```python
from build123d import *

# Parameters (mm, degrees)
F0_W     = 230.405122
F0_H     = 95.70128
F1_DEPTH = 25.4


with BuildPart() as f1:
    # F0 (on Front) → F1 (new body)
    with BuildSketch(Plane.XZ):
        Rectangle(F0_W, F0_H)
        Polygon((-70.301281, -22.45064), (-89.802561, -22.45064), (-89.802561, 2.94936), (-89.802561, 22.45064), (-70.301281, 22.45064), (-44.901281, 22.45064), (-19.501281, 22.45064), (19.501281, 22.45064), (44.901281, 22.45064), (70.301281, 22.45064), (89.802561, 22.45064), (89.802561, 2.94936), (89.802561, -22.45064), (64.402561, -22.45064), (25.4, -22.45064), (0, -22.45064), (-25.4, -22.45064), (-64.402561, -22.45064), align=None, mode=Mode.SUBTRACT)
        Polygon((-70.301281, 22.45064), (-70.301281, -22.45064), (-64.402561, -22.45064), (-44.901281, -2.94936), (-44.901281, 22.45064), align=None)
        Polygon((-44.901281, 22.45064), (-44.901281, -2.94936), (-25.4, -22.45064), (0, -22.45064), (0, 2.94936), (-19.501281, 22.45064), align=None)
        Polygon((0, 2.94936), (0, -22.45064), (25.4, -22.45064), (44.901281, -2.94936), (44.901281, 22.45064), (19.501281, 22.45064), align=None)
        Polygon((44.901281, 22.45064), (44.901281, -2.94936), (64.402561, -22.45064), (89.802561, -22.45064), (89.802561, 2.94936), (70.301281, 22.45064), align=None)
    extrude(amount=F1_DEPTH)


solid = f1.part
```
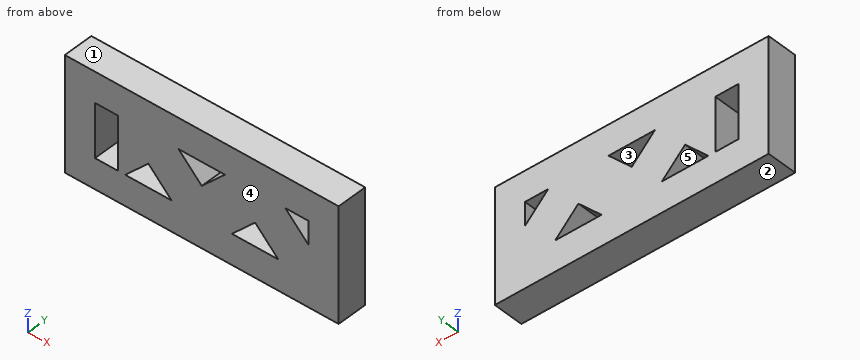
Geometry: final body of the model. Coordinates: model frame, mm. Face numbers are marked on the shaded views. A direction names the side the tool comes from. Round coordinates to 2 decimals unless told otherwise and drop trailing zeros. Order: outer loops, then holes, each group sorted by start corner. A loop starts at its lowest first (then second) coordinate and runs counter-clockwise, first axis right, second up. Notation, with made-up numbers: M 77,18.5 L 102,18.5 A17 ccw 102,37.5 Z; hole C 37.5,76.5 d6. An arc over 180 degrees is marked long. One line per item, written item: value.
(1) Cut plane D-D (x = -7). Return the cut outline in (y, z), and give its area (3 significant figures).
Result sheet:
outline: M -25.4,-47.85 L 0,-47.85 L 0,9.95 L -25.4,9.95 Z; M -25.4,22.45 L 0,22.45 L 0,47.85 L -25.4,47.85 Z
area: 2,110 mm2
(2) Pull-direction query (Z, two-part tool) for the marked faces 1, 2 and 3; classes: pulls with the +Z half, pulls with the -Z half, needs draft (parallel to the pull), parting line crosses it, or undercut.
Result sheet:
face 1: pulls with the +Z half
face 2: pulls with the -Z half
face 3: undercut
(3) Cut plane C-C (z = 10). Return the cut outline in (x, y).
Result sheet:
outline: M -115.2,-25.4 L -89.8,-25.4 L -89.8,0 L -115.2,0 Z; M -70.3,-25.4 L -7.05,-25.4 L -7.05,0 L -70.3,0 Z; M 7.05,-25.4 L 82.75,-25.4 L 82.75,0 L 7.05,0 Z; M 89.8,-25.4 L 115.2,-25.4 L 115.2,0 L 89.8,0 Z
(4) Cut plane B-B (y = -21). Return the cut outline in (x, z).
Result sheet:
outline: M -115.2,-47.85 L 115.2,-47.85 L 115.2,47.85 L -115.2,47.85 Z; hole M -89.8,-22.45 L -70.3,-22.45 L -70.3,22.45 L -89.8,22.45 Z; hole M -64.4,-22.45 L -25.4,-22.45 L -44.9,-2.95 Z; hole M -19.5,22.45 L 0,2.95 L 19.5,22.45 Z; hole M 25.4,-22.45 L 64.4,-22.45 L 44.9,-2.95 Z; hole M 70.3,22.45 L 89.8,2.95 L 89.8,22.45 Z
(5) Line query: probe 1 along X at (y, z) = (-20.5, -2.5); probe 2 along Z at (x, y) = (-76, -11.5); probe 3 along X at (y, z) = (-2.5, 10.5). Output: solid intervals per line, ascending. Write a range as [from, to].
Result sheet:
probe 1: [-115.2, -89.8], [-70.3, 115.2]
probe 2: [-47.85, -22.45], [22.45, 47.85]
probe 3: [-115.2, -89.8], [-70.3, -7.55], [7.55, 82.25], [89.8, 115.2]
(6) Reachability of the marked faces 4 and 5 from +Z, -Z, +X, -X, +Y, -Y: full face, straight path, thin tool, end or side. Return the list, or none.
Result sheet:
face 4: +Z, -Z, +X, -X, -Y
face 5: +Y, -Y
(7) Cut plane A-A (x = 38.5). Return the cut outline in (y, z), and give its area (3 significant figures).
Result sheet:
outline: M -25.4,-47.85 L 0,-47.85 L 0,-22.45 L -25.4,-22.45 Z; M -25.4,-9.35 L 0,-9.35 L 0,47.85 L -25.4,47.85 Z
area: 2,100 mm2
